```python
from build123d import *

# Parameters (mm, degrees)
F0_R     = 10
F0_R_2   = 3.2
F2_DEPTH = 13.5
F3_DEPTH = 25
F4_DEPTH = 11.4


with BuildPart() as f2:
    # F0 (on Top) → F2 (new body)
    with BuildSketch(Plane.XY):
        Circle(F0_R)
        Circle(F0_R_2, mode=Mode.SUBTRACT)
    extrude(amount=F2_DEPTH)

    # F1 (on Front) → F3 (cut)
    with BuildSketch(Plane.XZ):
        Polygon((-1, 10.25), (-1, 12.5), (-1, 15.121175), (-10.774387, 15.121175), (-10.774387, 12.5), (-10.774387, 10.25), (-3, 10.25), align=None)
        Polygon((1, 15.121175), (1, 12.5), (1, 10.25), (3, 10.25), (10.738912, 10.25), (10.738912, 12.5), (10.738912, 15.121175), align=None)
    extrude(amount=-F3_DEPTH, mode=Mode.SUBTRACT)

    # F1 (on Front) → F4 (cut)
    with BuildSketch(Plane.XZ):
        Polygon((-1, 10.25), (-1, 12.5), (-1, 15.121175), (-10.774387, 15.121175), (-10.774387, 12.5), (-10.774387, 10.25), (-3, 10.25), align=None)
        Polygon((1, 15.121175), (1, 12.5), (1, 10.25), (3, 10.25), (10.738912, 10.25), (10.738912, 12.5), (10.738912, 15.121175), align=None)
    extrude(amount=F4_DEPTH, mode=Mode.SUBTRACT)


solid = f2.part
```
Geometry: final body of the model. Coordinates: model frame, mm. A direction names the side the tool comes from. Give positions to 0.01 mm unless a question says otherwise; leave off trailing zeros. Loops run counter-clockwise (first coordinate to the right, second up) from the corner with the lowest first, then second, coordinate; pieces in that order, holes last. Notation, with made-up numbers: (31.5, 53.25) - (49.5, 53.25) arc R13 ccw to (49.5, 62.25) - close; hole circle Ø3 at (-39, 67). An arc over 180 degrees is marked (long way). Answer as CSV lines item,"result". Start each with the question number.
(1) Section query C-C (y = -8). Output: boundary loops of the cut face in (x, z).
(2) Reachability of faces 5 (the face through (1, 6, 12)), 6 (the face through (0, 7, 13.5)), 7 (the face through (-1, -6, 12)) from +Z, -Z, +X, -X, +Y, -Y: full face, straight path, thin tool, end or side. Return the list, or none.
(3) Ray query, line 1 along Y through (x, z) = (0, 5.25); line 2 along Z through (x, y) = (-1.25, 4.75). Return the intervals inside material, ascending. Write a range as [from, to].
(4) Pin query (flat end, axial travel): P1, Ø1.5, axis at x = 3.5, y = -7.5, coming from the +Z side; P2, Ø1.5, axis at y = 2.5, z = 4.5, coming from the -X side; P3, Ø2, axis at y = 6, z = 10, coming from the +X side. Return the tip coordinate at first contact, or that it passes through.
(5) Mould query, pull axis X, two halves, no side actions, for faces 1 (the face through (-3.2, 0.1, 5.2)), 2 (the face through (0, -6, 13.5)), 3 (the face through (-2.17, -9.76, 5.16)), 4 (the face through (1, -6, 12)). Classes: +X half, -X half, draft (parallel to the pull), parting line (faces both ways), or undercut.
(6) Section query B-B (z = 11.75). Output: boundary loops of the cut face in (x, y), and give its area (3 significant figures).
(7) Section query A-A (x = 0). Output: boundary loops of the cut face in (y, z).
(8) Section query D-D (z = 6.5). Output: boundary loops of the cut face in (x, y), and give its area (3 significant figures).
Worked answers:
1,outline,"(-6, 0) - (6, 0) - (6, 10.25) - (1, 10.25) - (1, 13.5) - (-1, 13.5) - (-1, 10.25) - (-6, 10.25) - close"
2,face 5,"+Z, +X, +Y, -Y"
2,face 6,"+Z, +X, -X, +Y, -Y"
2,face 7,"+Z, -X, +Y, -Y"
3,line 1,"y = [-10, -3.2], [3.2, 10]"
3,line 2,"z = [0, 10.25]"
4,P1,"stops at z = 10.25"
4,P2,"stops at x = -9.85"
4,P3,"stops at x = 8.66"
5,face 1,"undercut"
5,face 2,"draft"
5,face 3,"parting line"
5,face 4,"+X half"
6,outline,"(-1, -9.95) arc R10 ccw to (1, -9.95) - (1, -3.04) arc R3.2 cw to (-1, -3.04) - close; (-1, 3.04) arc R3.2 cw to (1, 3.04) - (1, 9.95) arc R10 ccw to (-1, 9.95) - close"
6,area,"27.3 mm^2"
7,outline,"(-10, 0) - (-3.2, 0) - (-3.2, 13.5) - (-10, 13.5) - close; (3.2, 0) - (10, 0) - (10, 13.5) - (3.2, 13.5) - close"
8,outline,"circle Ø20 at (0, 0); hole circle Ø6.4 at (0, 0)"
8,area,"282 mm^2"
